Could you check a few things on this drawing? It's one solid part, dimensions in mm from its lowest x, y, z. A direction names the side the tool comes from. Round coordinates to 2 decimals unless told otherwise and drop trailing zeros. Write each loop counter-clockwise with the first axis right and the second up, starting at its lowest first coordinate (ties: lowest second). Pieces come first, ordered by that corner, then holes. Notation, with made-up numbers: (-3, 11) -> (52, 11) arc R27 cw to (52, 48) -> close; hole circle Ø6 at (-8.75, 34). An arc over 180 degrees is marked (long way). Return JSON: item names as keys, results as strings.
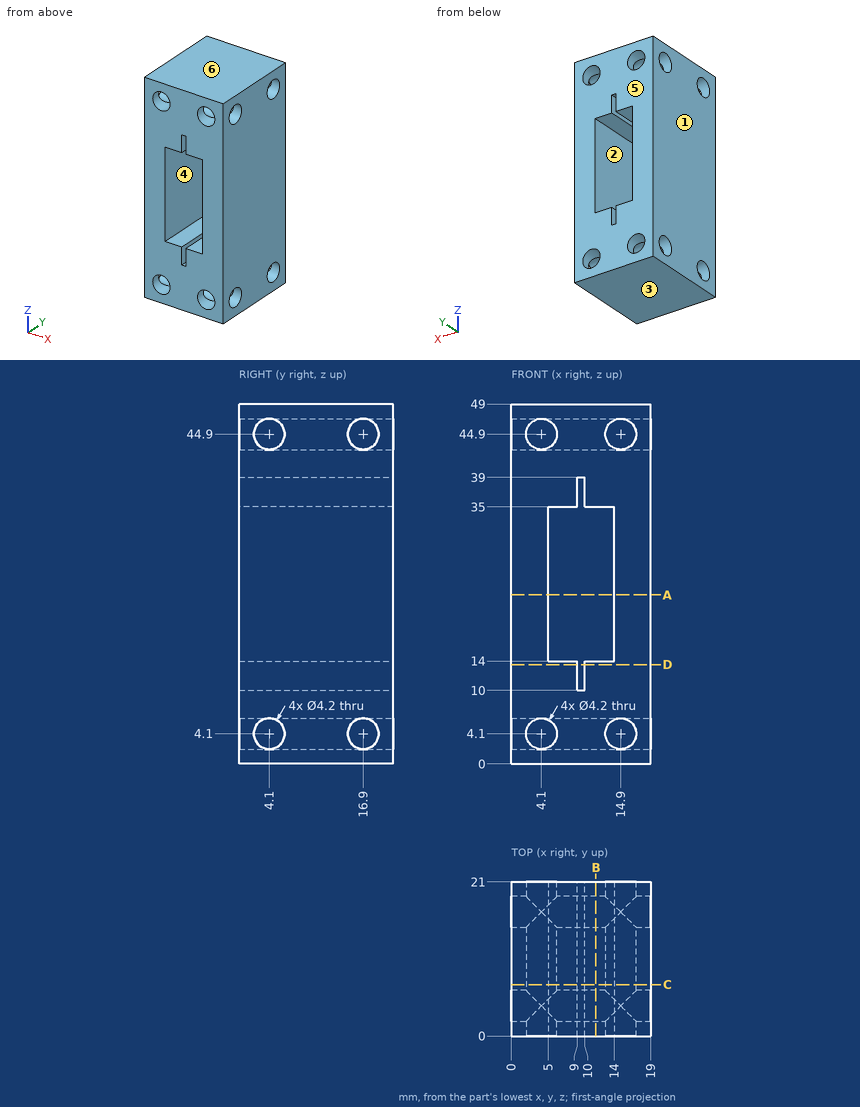
1) I want a section at D-D, the plane z = 13.5. Please give me the cut outline in (x, y).
Return value:
{"outline": "(0, 0) -> (9, 0) -> (9, 21) -> (0, 21) -> close; (10, 0) -> (19, 0) -> (19, 21) -> (10, 21) -> close"}
2) I want a section at A-A, the plane z = 23. Please give me the cut outline in (x, y), and give its area (3 significant figures).
Return value:
{"outline": "(0, 0) -> (5, 0) -> (5, 21) -> (0, 21) -> close; (14, 0) -> (19, 0) -> (19, 21) -> (14, 21) -> close", "area": "210 mm²"}
3) I want a section at C-C, the plane y = 7. Please give me the cut outline in (x, z).
Return value:
{"outline": "(0, 0) -> (19, 0) -> (19, 49) -> (0, 49) -> close; hole circle Ø4.2 at (4.1, 4.1); hole circle Ø4.2 at (4.1, 44.9); hole (5, 14) -> (9, 14) -> (9, 10) -> (10, 10) -> (10, 14) -> (14, 14) -> (14, 35) -> (10, 35) -> (10, 39) -> (9, 39) -> (9, 35) -> (5, 35) -> close; hole circle Ø4.2 at (14.9, 4.1); hole circle Ø4.2 at (14.9, 44.9)"}
4) Thinking about a two-plate mould opening in Z: for the marked faces 3, 4, 5 and 6, which applies, pulls with the +Z half, pulls with the -Z half, needs draft (parallel to the pull), parting line crosses it, or undercut?
Return value:
{"face 3": "pulls with the -Z half", "face 4": "undercut", "face 5": "needs draft", "face 6": "pulls with the +Z half"}
5) If I drill on probe 1 along Y at (x, z) = (8, 4.1); probe 2 along Z at (x, y) = (14.9, 1.85); probe 3 along Z at (x, y) = (8, 14.5), over which ranges is the centre line in solid material (lowest first)? Write a range as [from, to].
Return value:
{"probe 1": "[0, 2], [6.2, 14.8], [19, 21]", "probe 2": "[0, 2], [6.2, 42.8], [47, 49]", "probe 3": "[0, 14], [35, 49]"}
6) I want a section at B-B, the plane x = 11.5. Please give me the cut outline in (y, z).
Return value:
{"outline": "(0, 0) -> (21, 0) -> (21, 14) -> (0, 14) -> close; (0, 35) -> (21, 35) -> (21, 49) -> (0, 49) -> close; hole circle Ø4.2 at (4.1, 4.1); hole circle Ø4.2 at (4.1, 44.9); hole circle Ø4.2 at (16.9, 4.1); hole circle Ø4.2 at (16.9, 44.9)"}
7) For the marked faces 1 and 2, which set-ups out of +Z, -Z, +X, -X, +Y, -Y let a thin tool reach every point of the face, with its end or its side?
Return value:
{"face 1": "+Z, -Z, -X, +Y, -Y", "face 2": "+Y, -Y"}
8) Will this pin go through, and if not, where does the flat tip stop? pin 1 Ø6.5 at (y, z) = (4.1, 44.9) entering from -X.
Return value:
{"pin 1": "x = 0"}
